Verification items for the finished model (mm, model axes). Face numbers are marked on the shaded views. Give positions to 0.01 mm unless a question says otherwise; leave off trailing zeros. Write each loop counter-clockwise with the first axis right and the second up, starting at its lowest first coordinate (ties: lowest second). Pieces come first, ordered by that corner, then holes. Notation, with made-up numbers: (14, -20) -> (30, -20) arc R24 cw to (30, 6) -> close; hole circle Ø2 at (14, 63). An arc over 180 degrees is marked (long way). Use one line per item in the form item = value. Start each with the question number.
(1) Section check C-C, the plane x = -37.5. Record the cut outline in (y, z), plus the area to 3 significant figures.
(2) Scan lines: L1, parallel to X at y = -5, z = 0.9; L2, parallel to X at y = -25.87, z = 3.3; L3, parallel to Y at x = 6.25, z = 1.9. Record each from-to range of solid material in increasing order.
(3) Section check B-B, the plane y = -25.87. Record the cut outline in (x, z).
(4) Section check A-A, the plane x = 17.5. Record the cut outline in (y, z), plus the area to 3 significant figures.
(5) Release check for a two-part mould opening along X. For the marked faces 1 and 2 record: pulls with the +X half, pulls with the -X half, needs draft (parallel to the pull), parting line crosses it, or undercut.
(6) Section check D-D, the plane x = -6.25. Record the cut outline in (y, z), plus the area to 3 significant figures.
(7) Depth check by flat-ended pin: pin 1 Ø1.2 at (y, z) = (-4.5, 2.5) entering from +X; pin 2 Ø3 at (y, z) = (-10.5, 2.5) entering from +X; pin 3 Ø4 at (x, y) = (37.5, -15) entering from +Z. Enter the tip coordinate at first touch or a pass-through.
Solid Edge part; units mm, degrees
sketch "Sketch1" plane through (0, 0, 0) normal (0, 0, 1) x (1, 0, 0)
  line L0 (0, 0) -> (-25, 0)
  line L1 (-25, 0) -> (-25, -8.58)
  line L2 (-25, -8.58) -> (-55.28, -8.58)
  line L3 (-55.28, -8.58) -> (-40, -20)
  line L4 (-40, -20) -> (-40, -40.11)
  line L5 (-40, -40.11) -> (0, -40.11)
  line L6 (0, -40.11) -> (0, 0)
  dimension "D1" = 40
  dimension "D2" = 25
  dimension "D3" = 25
extrude "Protrusion1" add sketch "Sketch1" along normal blind 5
mirror "Mirror1" about plane through (0, 0, 0) normal (1, 0, 0) of "Protrusion1"
chamfer "Fase_1" distance 1 angle 45 10 edges at (-40.14, -8.58, 5) (-25, -4.29, 5) (0, 0, 5) (25, -4.29, 5) (40.14, -8.58, 5) (47.64, -14.29, 5) (40, -30.055, 5) (0, -40.11, 5) (-40, -30.055, 5) (-47.64, -14.29, 5)
sketch "Sketch2" plane through (0, -20.055, 5) normal (0, 0, 1) x (1, 0, 0)
  circle A0 centre (-25, 5.055) radius 2.65
  circle A1 centre (25, 5.055) radius 2.65
  dimension "D1" = 25
extrude "Extrusionsausschnitt_1" cut sketch "Sketch2" against normal blind 40
sketch "Sketch3" plane through (0, -20.055, 5) normal (0, 0, 1) x (1, 0, 0)
  line L0 (-15.9123, 17.805) -> (-19.0877, 17.805)
  line L1 (-19.0877, 17.805) -> (-20.6754, 15.055)
  line L2 (-20.6754, 15.055) -> (-19.0877, 12.305)
  line L3 (-19.0877, 12.305) -> (-15.9123, 12.305)
  line L4 (-15.9123, 12.305) -> (-14.3246, 15.055)
  line L5 (-14.3246, 15.055) -> (-15.9123, 17.805)
  line L6 (19.0877, 17.805) -> (15.9123, 17.805)
  line L7 (15.9123, 17.805) -> (14.3246, 15.055)
  line L8 (14.3246, 15.055) -> (15.9123, 12.305)
  line L9 (15.9123, 12.305) -> (19.0877, 12.305)
  line L10 (19.0877, 12.305) -> (20.6754, 15.055)
  line L11 (20.6754, 15.055) -> (19.0877, 17.805)
  line L12 (39.0877, 7.805) -> (35.9123, 7.805)
  line L13 (35.9123, 7.805) -> (34.3246, 5.055)
  line L14 (34.3246, 5.055) -> (35.9123, 2.305)
  line L15 (35.9123, 2.305) -> (39.0877, 2.305)
  line L16 (39.0877, 2.305) -> (40.6754, 5.055)
  line L17 (40.6754, 5.055) -> (39.0877, 7.805)
  line L18 (-35.9123, 7.805) -> (-39.0877, 7.805)
  line L19 (-39.0877, 7.805) -> (-40.6754, 5.055)
  line L20 (-40.6754, 5.055) -> (-39.0877, 2.305)
  line L21 (-39.0877, 2.305) -> (-35.9123, 2.305)
  line L22 (-35.9123, 2.305) -> (-34.3246, 5.055)
  line L23 (-34.3246, 5.055) -> (-35.9123, 7.805)
extrude "Extrusionsausschnitt_2" cut sketch "Sketch3" against normal blind 2.5
hole "Bohrung_1" at (-37.5, -15, 2.5) direction (0, 0, -1) diameter 3.6 end up to next
hole "Hole1" at (-17.5, -5, 2.5) direction (0, 0, -1) diameter 3.6 end up to next
hole "Hole2" at (17.5, -5, 2.5) direction (0, 0, -1) diameter 3.6 end up to next
hole "Hole3" at (37.5, -15, 2.5) direction (0, 0, -1) diameter 3.6 end up to next
hole "Bohrung_5" at (-6.25, -25.87, 5) direction (0, 0, -1) diameter 5.8 end up to next
hole "Hole4" at (6.25, -25.87, 5) direction (0, 0, -1) diameter 5.8 end up to next
properties part number "50" material "Polyacticacid"
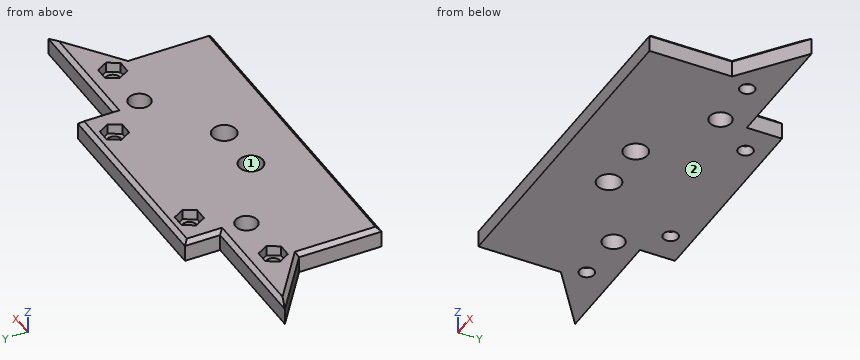
Completed:
q1.outline = (-40.11, 0) -> (-16.8, 0) -> (-16.8, 2.5) -> (-17.75, 2.5) -> (-17.75, 5) -> (-39.11, 5) -> (-40.11, 4) -> close; (-13.2, 0) -> (-8.58, 0) -> (-8.58, 4) -> (-9.58, 5) -> (-12.25, 5) -> (-12.25, 2.5) -> (-13.2, 2.5) -> close
q1.area = 134 mm²
q2.L1 = -25 to -19.3, -15.7 to 15.7, 19.3 to 25
q2.L2 = -40 to -9.15, -3.35 to 3.35, 9.15 to 40
q2.L3 = -40.11 to -28.77, -22.97 to 0
q3.outline = (-40, 0) -> (-9.15, 0) -> (-9.15, 5) -> (-39, 5) -> (-40, 4) -> close; (-3.35, 0) -> (3.35, 0) -> (3.35, 5) -> (-3.35, 5) -> close; (9.15, 0) -> (40, 0) -> (40, 4) -> (39, 5) -> (9.15, 5) -> close
q4.outline = (-40.11, 0) -> (-6.8, 0) -> (-6.8, 2.5) -> (-7.75, 2.5) -> (-7.75, 5) -> (-39.11, 5) -> (-40.11, 4) -> close; (-3.2, 0) -> (0, 0) -> (0, 4) -> (-1, 5) -> (-2.25, 5) -> (-2.25, 2.5) -> (-3.2, 2.5) -> close
q4.area = 177 mm²
q5.face_1 = undercut
q5.face_2 = needs draft
q6.outline = (-40.11, 0) -> (-28.77, 0) -> (-28.77, 5) -> (-39.11, 5) -> (-40.11, 4) -> close; (-22.97, 0) -> (0, 0) -> (0, 4) -> (-1, 5) -> (-22.97, 5) -> close
q6.area = 171 mm²
q7.pin_1 = 25
q7.pin_2 = 54.72
q7.pin_3 = 2.5
